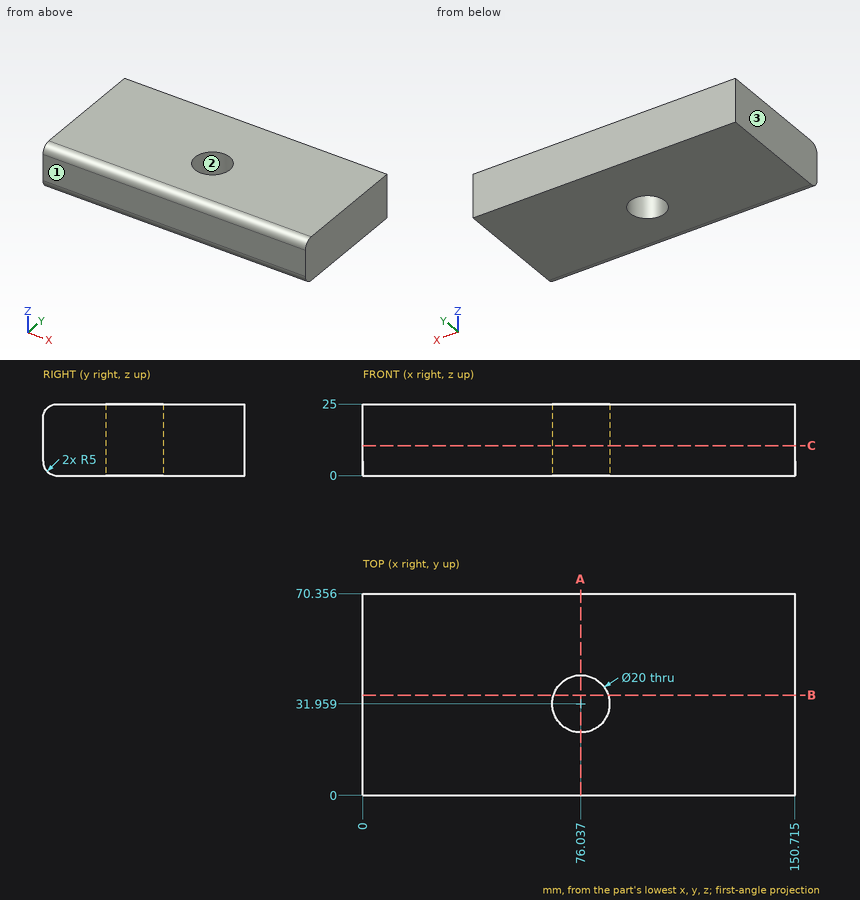
Source: three-view drawing plus pictorial views. Frame: mm from the lowest corner of the part. Coordinates: 2 decimals unless noted, no trailing zeros. Write each loop counter-clockwise with the first axis right and the second up, starting at its lowest first coordinate (ties: lowest second). Pieces come first, ordered by that corner, then holes. Notation, with made-up numbers: (51, -37.75) -> (91, -37.75) arc R16 ccw to (91, -6.75) -> close; hole circle Ø11 at (13.25, 83). An arc over 180 degrees is marked (long way). Answer as a JSON object with one key per item and string values.
1. Mould query, pull axis X, two halves, no side actions, for the marked faces 1, 2 and 3. Classes: released by +X, released by -X, zero draft, split by the parting line, or undercut.
Result set:
{"face 1": "zero draft", "face 2": "undercut", "face 3": "released by -X"}
2. Material intervals for line 1 (X direction, y = 25, z = 10.25) (1 decimal); line 2 (X direction, y = 24, z = 12) (1 decimal); line 3 (Y direction, x = 69, z = 23) (1 decimal), sorted ascending. Write a range as from..to.
Result set:
{"line 1": "x = 0..68.9, 83.2..150.7", "line 2": "x = 0..70, 82.1..150.7", "line 3": "y = 1..24.9, 39.1..70.4"}
3. First-contact query: P1, Ø6, axis at y = 14.5, z = 19, coming from the -X side. Flat tip, straight axial feed; report the tip coordinate or a pass-through.
Result set:
{"P1": "stops at x = 0"}
4. Section C-C on z = 10.5. Return the cut outline in (x, y) (1 decimal).
Result set:
{"outline": "(0, 0) -> (150.7, 0) -> (150.7, 70.4) -> (0, 70.4) -> close; hole circle Ø20 at (76, 32)"}
5. Section A-A on x = 76. Return the cut outline in (y, z).
Result set:
{"outline": "(0, 5) arc R5 ccw to (5, 0) -> (21.96, 0) -> (21.96, 25) -> (5, 25) arc R5 ccw to (0, 20) -> close; (41.96, 0) -> (70.36, 0) -> (70.36, 25) -> (41.96, 25) -> close"}
6. Section B-B on y = 35. Return the cut outline in (x, z) (1 decimal), then the cut area to 3 significant figures.
Result set:
{"outline": "(0, 0) -> (66.5, 0) -> (66.5, 25) -> (0, 25) -> close; (85.6, 0) -> (150.7, 0) -> (150.7, 25) -> (85.6, 25) -> close", "area": "3,290 mm2"}
